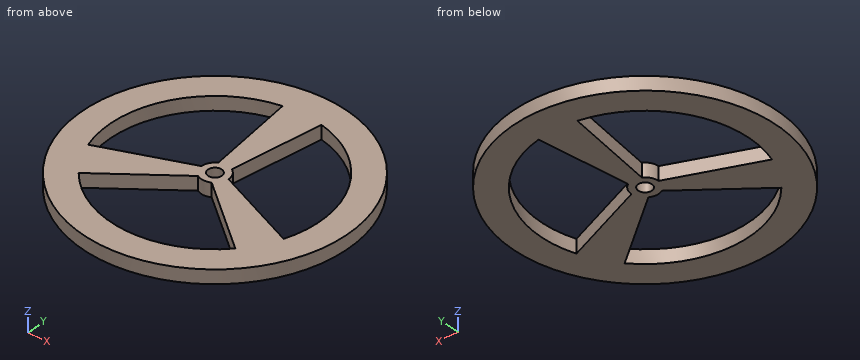
```python
from build123d import *

# Parameters (mm, degrees)
SKETCH1_R           = 48.1
SKETCH1_R_2         = 2.5
BOSS_EXTRUDE1_DEPTH = 5


with BuildPart() as part:
    # Sketch1 → Boss-Extrude1 (new body)
    with BuildSketch(Plane.XY):
        Circle(SKETCH1_R)
        with BuildLine():
            Line((-7.150888472, 37.422918032), (-2.5, 4.330127019))
            ThreePointArc((-2.5, 4.330127019), (-4.330127019, 2.5), (-5, 0))
            Line((-5, 0), (-35.984641936, -12.51860794))
            ThreePointArc((-35.984641936, -12.51860794), (-32.995567884, 19.05), (-7.150888472, 37.422918032))
        make_face(mode=Mode.SUBTRACT)
        with BuildLine():
            Line((-28.833753464, -24.904310092), (-2.5, -4.330127019))
            ThreePointArc((-2.5, -4.330127019), (0, -5), (2.5, -4.330127019))
            Line((2.5, -4.330127019), (28.833753464, -24.904310092))
            ThreePointArc((28.833753464, -24.904310092), (0, -38.1), (-28.833753464, -24.904310092))
        make_face(mode=Mode.SUBTRACT)
        with BuildLine():
            Line((35.984641936, -12.51860794), (5, 0))
            ThreePointArc((5, 0), (4.330127019, 2.5), (2.5, 4.330127019))
            Line((2.5, 4.330127019), (7.150888472, 37.422918032))
            ThreePointArc((7.150888472, 37.422918032), (32.995567884, 19.05), (35.984641936, -12.51860794))
        make_face(mode=Mode.SUBTRACT)
        Circle(SKETCH1_R_2, mode=Mode.SUBTRACT)
    extrude(amount=BOSS_EXTRUDE1_DEPTH)


solid = part.part
```
Read the model definition and answer for the solid it produces. Units are mm, in the model's axes. Give positions to 0.01 mm unless a question says otherwise; leave off trailing zeros. Order: outer loops, then holes, each group sorted by start corner. A loop starts at its lowest first (then second) coordinate and runs counter-clockwise, first axis right, second up. Notation, with made-up numbers: (-13.75, -9.5) -> (21.25, -9.5) arc R18 cw to (21.25, 10.5) -> close; hole circle Ø11 at (-21, 87.25). An arc over 180 degrees is marked (long way). One line per item, written item: value. Start each with the question number.
(1) The part is cut by section B-B (y = -8). Determine the outline of the cut face in (x, z).
(2) The part is cut by section A-A (x = 0). Determine the outline of the cut face in (y, z).
(3) Flat-ended cylindrical pins translate along their axes: P1, Ø2, axis at x = -22, z = 1, coming from the -Y side; P2, Ø4, axis at x = -37.5, y = 20, coming from the -Z side; P3, Ø1.5, axis at x = 13.5, z = 2, coming from the -Y side; P4, Ø4.5, axis at x = 0, y = 0, coming from the -Z side. Find the tip coordinate at first contact, or state that the pin passes through.
(4) The part is cut by section C-C (z = 2.7). Determine the outline of the cut face in (x, y).
(5) The part is cut by section D-D (x = 33). Determine the outline of the cut face in (y, z), and give its area (3 significant figures).
(6) Straight lines are drawn through the part: L1, parallel to Y at x = 0, z = 2.55; L2, parallel to X at y = 19, z = 4.5; L3, parallel to X at y = 25.5, z = 1.3. For each, find the intervals that lie inside material, in ascending order.
Taken from the geometry:
1. outline: (-47.43, 0) -> (-37.25, 0) -> (-37.25, 5) -> (-47.43, 5) -> close; (-24.8, 0) -> (-7.2, 0) -> (-7.2, 5) -> (-24.8, 5) -> close; (7.2, 0) -> (24.8, 0) -> (24.8, 5) -> (7.2, 5) -> close; (37.25, 0) -> (47.43, 0) -> (47.43, 5) -> (37.25, 5) -> close
2. outline: (-48.1, 0) -> (-38.1, 0) -> (-38.1, 5) -> (-48.1, 5) -> close; (-5, 0) -> (-2.5, 0) -> (-2.5, 5) -> (-5, 5) -> close; (2.5, 0) -> (48.1, 0) -> (48.1, 5) -> (2.5, 5) -> close
3. P1: y = -43.27
3. P2: z = 0
3. P3: y = -46.38
3. P4: through
4. outline: circle Ø96.2 at (0, 0); hole (-35.98, -12.52) -> (-5, 0) arc R5 cw to (-2.5, 4.33) -> (-7.15, 37.42) arc R38.1 ccw to start; hole (-28.83, -24.9) arc R38.1 ccw to (28.83, -24.9) -> (2.5, -4.33) arc R5 cw to (-2.5, -4.33) -> close; hole circle Ø5 at (0, 0); hole (2.5, 4.33) arc R5 cw to (5, 0) -> (35.98, -12.52) arc R38.1 ccw to (7.15, 37.42) -> close
5. outline: (-34.99, 0) -> (-11.31, 0) -> (-11.31, 5) -> (-34.99, 5) -> close; (19.04, 0) -> (34.99, 0) -> (34.99, 5) -> (19.04, 5) -> close
5. area: 198 mm^2
6. L1: -48.1 to -38.1, -5 to -2.5, 2.5 to 48.1
6. L2: -44.19 to -33.02, -4.56 to 4.56, 33.02 to 44.19
6. L3: -40.78 to -28.31, -5.48 to 5.48, 28.31 to 40.78
